Geometry check sheet. Reference: the model listing, model coordinates, mm. Give positions to 0.01 mm unless a question says otherwise; leave off trailing zeros. Write each loop counter-clockwise with the first axis right and the second up, starting at its lowest first coordinate (ties: lowest second). Pieces come first, ordered by that corner, then holes. Notation, with made-up numbers: M 54.5,-18.5 L 62.5,-18.5 A10 ccw 62.5,-11.5 Z; hole C 63,-23.5 d4. An arc over 180 degrees is marked long. Write each question's results on one line, items separated by ' | '.
```python
from build123d import *

# Parameters (mm, degrees)
SKETCH1_R           = 6
BOSS_EXTRUDE1_DEPTH = 45
SKETCH2_R           = 2.1
CUT_EXTRUDE1_DEPTH  = 46
SKETCH5_R           = 2.5
CUT_EXTRUDE2_DEPTH  = 22.5


with BuildPart() as part:
    # Sketch1 → Boss-Extrude1 (new body)
    with BuildSketch(Plane.XY):
        Circle(SKETCH1_R)
    extrude(amount=BOSS_EXTRUDE1_DEPTH)

    # Sketch2 → Cut-Extrude1 (cut, through all)
    with BuildSketch(Plane.XY.offset(45)):
        Circle(SKETCH2_R)
    extrude(amount=-CUT_EXTRUDE1_DEPTH, mode=Mode.SUBTRACT)

    # Sketch5 → Cut-Extrude2 (cut, symmetric)
    with BuildSketch(Plane.XY.offset(45)):
        Circle(SKETCH5_R)
    extrude(amount=CUT_EXTRUDE2_DEPTH, both=True, mode=Mode.SUBTRACT)


solid = part.part
```
Q1. Release check for a two-part mould opening along Y. For faces 1 (the face through (-6, 0, 22)), 2 (the face through (2.003, 0.631, 11.407)), 3 (the face through (-0.54, -2.44, 33.91)), 4 (the face through (3, 0, 45)) record: released by +Y, released by -Y, zero draft, split by the parting line, or undercut.
Answer key:
face 1: split by the parting line | face 2: undercut | face 3: undercut | face 4: zero draft
Q2. Section check C-C (z = 11). Enter the section's corners in (x, y), then the cut area to 3 significant figures.
Answer key:
outline: C 0,0 d12; hole C 0,0 d4.2 | area: 99.2 mm2
Q3. Section check A-A (x = 0). Enter the section's corners in (y, z).
Answer key:
outline: M -6,0 L -2.1,0 L -2.1,22.5 L -2.5,22.5 L -2.5,45 L -6,45 Z; M 2.1,0 L 6,0 L 6,45 L 2.5,45 L 2.5,22.5 L 2.1,22.5 Z
Q4. Depth check by flat-ended pin: P1, Ø6, axis at x = 1.5, y = -1.5, coming from the +Z side; P2, Ø1, axis at y = 4, z = 11.5, coming from the +X side; P3, Ø1, axis at x = 2.5, z = 31, coming from the +Y side. Enter the tip coordinate at first touch or a pass-through.
Answer key:
P1: stops at z = 45 | P2: stops at x = 4.87 | P3: stops at y = 5.66
Q5. Material ranges on probe 1 along Y at (x, z) = (0, 12); probe 2 along Y at (x, z) = (0, 37.75); probe 3 along X at (y, z) = (1, 21.5), recorded low to high. Write a range as [from, to].
Answer key:
probe 1: y = [-6, -2.1], [2.1, 6] | probe 2: y = [-6, -2.5], [2.5, 6] | probe 3: x = [-5.92, -1.85], [1.85, 5.92]
Q6. Section check D-D (x = 4.5). Enter the section's corners in (y, z), then the cut area to 3 significant figures.
Answer key:
outline: M -3.97,0 L 3.97,0 L 3.97,45 L -3.97,45 Z | area: 357 mm2
